Here's the drawing with two shaded views (mm, measured from the low corner). I have some questions. Round coordinates to 2 decimals unless told otherwise and drop trailing zeros. Write each loop counter-clockwise with the first axis right and the second up, starting at its lowest first coordinate (ties: lowest second). Pieces come first, ordered by that corner, then holes. Notation, with made-up numbers: M 66.25,32.5 L 87.25,32.5 A18 ccw 87.25,57.5 Z; hole C 61,-33.5 d8. An arc over 180 degrees is marked long. Answer as a JSON object with one key per item and string values. Group by question number.
1) Suppose I cut it at C-C, the plane z = 3.75. Write out the boundary of the cut face in (x, y), and give its area (3 significant figures).
2) Please list where these lines run through material, in increasing order: L1, parallel to X at y = 1.4, z = 1.5; L2, parallel to Z at x = 14.25, y = 1.3; L3, parallel to Y at x = 20.5, z = 8. Write a range as [from, to].
3) If we mould it in two halves opening along X, with no side actions, what happens to the marked faces 1, 2 and 3? For each: +X half, -X half, draft (parallel to the pull), parting line (faces both ways), or undercut.
4) Suppose I cut it at B-B, the plane x = 4.5. Write out the boundary of the cut face in (y, z).
5) Suppose I cut it at A-A, the plane y = 1.8. Write out the boundary of the cut face in (x, z), and give its area (3 significant figures).
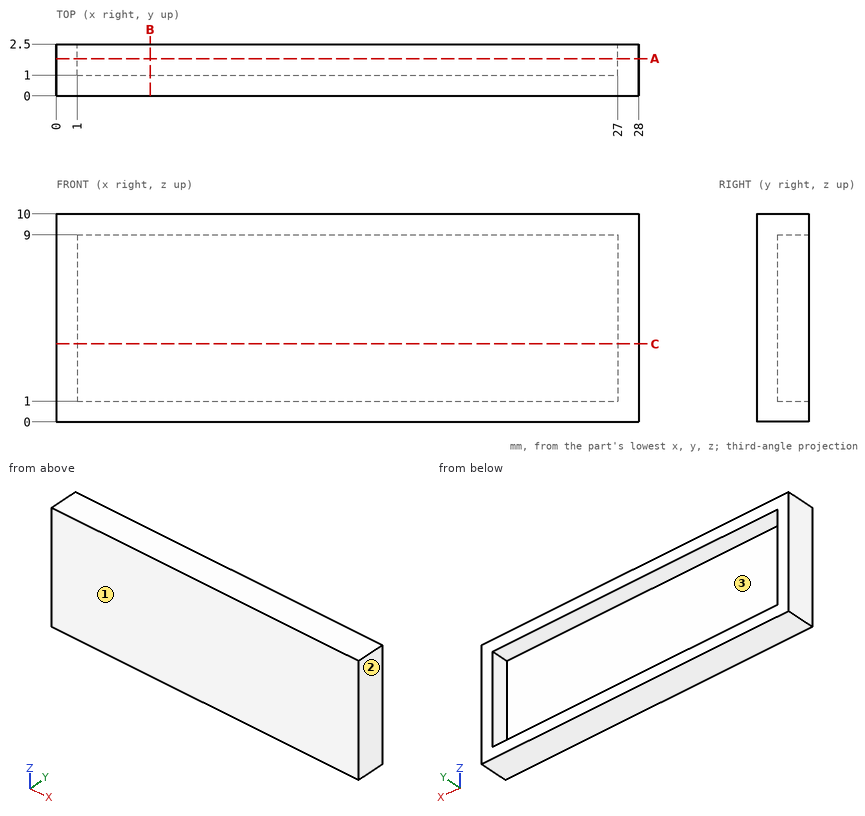
Results:
{
 "1": {"outline": "M 0,0 L 28,0 L 28,2.5 L 27,2.5 L 27,1 L 1,1 L 1,2.5 L 0,2.5 Z", "area": "31.0 mm^2"},
 "2": {"L1": "[0, 1], [27, 28]", "L2": "[0, 1], [9, 10]", "L3": "[0, 1]"},
 "3": {"face 1": "draft", "face 2": "+X half", "face 3": "undercut"},
 "4": {"outline": "M 0,0 L 2.5,0 L 2.5,1 L 1,1 L 1,9 L 2.5,9 L 2.5,10 L 0,10 Z"},
 "5": {"outline": "M 0,0 L 28,0 L 28,10 L 0,10 Z; hole M 1,1 L 27,1 L 27,9 L 1,9 Z", "area": "72.0 mm^2"}
}
